Autodesk Inventor part; units mm, degrees
ref_plane "YZ Plane" through (0, 0, 0) normal (1, 0, 0) x (0, 1, 0)
ref_plane "XZ Plane" through (0, 0, 0) normal (0, 1, 0) x (-1, 0, 0)
ref_plane "XY Plane" through (0, 0, 0) normal (0, 0, 1) x (1, 0, 0)
sketch "Эскиз1" plane through (0, 0, 0) normal (0, 1, 0) x (-1, 0, 0)
  line L0 (43.5, -29.5) -> (-43.5, -29.5)
  line L1 (-43.5, -29.5) -> (-43.5, 29.5)
  line L2 (-43.5, 29.5) -> (43.5, 29.5)
  line L3 (43.5, 29.5) -> (43.5, -29.5)
  line L4 (43.5, -29.5) -> (-43.5, 29.5) construction
  line L5 (-43.5, -29.5) -> (43.5, 29.5) construction
  point P0 (0, 0)
  dimension "d0" = 87
  dimension "d1" = 59
extrude "Выдавливание1" add sketch "Эскиз1" along normal blind 2
sketch "Эскиз2" plane through (0, 2, 0) normal (0, 1, 0) x (1, 0, 0)
  line L0 (43.5, -28) -> (-43.5, -28)
  line L1 (-43.5, -28) -> (-43.5, 28)
  line L2 (-43.5, 28) -> (43.5, 28)
  line L3 (43.5, 28) -> (43.5, -28)
  line L4 (43.5, -28) -> (-43.5, 28) construction
  line L5 (-43.5, -28) -> (43.5, 28) construction
  point P0 (0, 0)
  dimension "d4" = 87
  dimension "d5" = 56
extrude "Выдавливание2" add sketch "Эскиз2" along normal blind 3
sketch "Эскиз3" plane through (0, 0, 0) normal (0, -1, 0) x (1, 0, 0)
  line L0 (43.5, 29.5) -> (43.5, -29.5)
  line L1 (43.5, 0) -> (43.5, -30.5)
  line L2 (43.5, 0) -> (43.5, 30.5)
  line L3 (43.5, -30.5) -> (43.5, -27.5)
  circle A0 centre (43.5, -27.5) radius 3
  line L4 (43.5, 0) -> (-8.3438, 0)
  circle A1 centre (43.5, 27.5) radius 3
  line L5 (46.5, 27.5) -> (46.5, -27.5)
  point P0 (0, 0)
  dimension "d8" = 30.5
  dimension "d9" = 30.5
  dimension "d10" = 3
extrude "Выдавливание3" add sketch "Эскиз3" against normal blind 5 contours L0 A0 L1 | L0 A1 L5 A0 | L0 L2 A1 picked at (44.2818, -28.7902) picked at (43.7225, 26.1917)
properties part number "bt-lid"
Could you check a few things on this model? Use its own coordinates, in mm. A direction names the side the tool comes from. Coordinates: 2 decimals unless noted, no trailing zeros. Order: outer loops, then holes, each group sorted by start corner. A loop starts at its lowest first (then second) coordinate and runs counter-clockwise, first axis right, second up. Notation, with made-up numbers: M 62.5,19 L 115.5,19 A17 ccw 115.5,46 Z; hole C 50,4 d9. An arc over 180 degrees is marked long. Use a Markdown table: item, result. Add a question column.
Q1. Which directions (+Z, -Z, +X, -X, +Y, -Y) give clear straight access to the entire face, cutting with the end or side of a thin tool? Please do faces 1 (the flat face through (-1, 3, -28)), 2 (the flat face through (1, 1, 29.5)), 3 (the flat face through (1, 0, 0)), 4 (the flat face through (1, 3, 28)), 5 (the flat face through (-1, 1, -29.5)).
Q2. I want a section at A-A on y = 3.45. List the corners of the cut face in (x, z) for me.
Q3. I'm going to push flat-ended pins straight in: pin 1 (1.2 mm diameter, centred on x = 20.5, z = 29, fed in from +Y); pin 2 (0.6 mm diameter, centred on x = 2.5, y = 1, fed in from -Z); pin 3 (1.5 mm diameter, centred on x = -11.5, y = 3, fed in from -Z). Where does each tip first touch, or does it pass through?
Q4. I want a section at B-B on x = -0.5. List the corners of the cut face in (y, z) for me.
Q5. If I drill on L1, parallel to Z at x = -1, y = 2.15; L2, parallel to Z at x = -9, y = 0.75, over which ranges is the centre line in solid material (lowest first)?
Checked values:
| question | item | result |
|---|---|---|
| 1 | face 1 | -Z, -X, +Y |
| 1 | face 2 | +Z, -X, +Y, -Y |
| 1 | face 3 | +Z, -Z, +X, -X, -Y |
| 1 | face 4 | +Z, -X, +Y |
| 1 | face 5 | -Z, -X, +Y, -Y |
| 2 | outline | M -43.5,-28 L 43.5,-28 L 43.5,-30.5 A3 ccw 46.5,-27.5 L 46.5,27.5 A3 ccw 43.5,30.5 L 43.5,28 L -43.5,28 Z |
| 3 | pin 1 | y = 2 |
| 3 | pin 2 | z = -29.5 |
| 3 | pin 3 | z = -28 |
| 4 | outline | M 0,-29.5 L 2,-29.5 L 2,-28 L 5,-28 L 5,28 L 2,28 L 2,29.5 L 0,29.5 Z |
| 5 | L1 | -28 to 28 |
| 5 | L2 | -29.5 to 29.5 |
